```python
from build123d import *

# Parameters (mm, degrees)
F0_R     = 20.05
F1_DEPTH = 3.1
F2_R     = 10.05
F3_DEPTH = 2
F4_R     = 0.5
F5_R     = 2.5
F6_DEPTH = 3.1010001
F7_W     = 1
F7_H     = 5
F8_DEPTH = 3.1010001


with BuildPart() as f1:
    # F0 (on Top) → F1 (new body)
    with BuildSketch(Plane.XY):
        Circle(F0_R)
    extrude(amount=F1_DEPTH)

    # F2 (on face) → F3 (cut)
    with BuildSketch(Plane.XY.offset(3.1)):
        with Locations((5, 0)):
            Circle(F2_R)
    extrude(amount=-F3_DEPTH, mode=Mode.SUBTRACT)

    # F4
    f4_edges = [f1.edges().sort_by_distance(p)[0] for p in [
        (-20.05, 0, 3.1),
        (-5.05, 0, 3.1),
        (-20.05, 0, 0),
    ]]
    fillet(f4_edges, radius=F4_R)

    # F5 (on face) → F6 (cut, through all)
    with BuildSketch(Plane(origin=(0, 0, 0), x_dir=(1, 0, 0), z_dir=(0, 0, -1))):
        Circle(F5_R)
    extrude(amount=-F6_DEPTH, mode=Mode.SUBTRACT)

    # F7 (on face) → F8 (cut, through all)
    with BuildSketch(Plane.XY.offset(3.1)):
        with Locations((0, 18.05)):
            Rectangle(F7_W, F7_H)
        with Locations((0, -18.05)):
            Rectangle(F7_W, F7_H)
    extrude(amount=-F8_DEPTH, mode=Mode.SUBTRACT)


solid = f1.part
```
CAD build for the part. Positions are in the model's coordinates, mm. A direction names the side the tool comes from. Round coordinates to 2 decimals unless told otherwise and drop trailing zeros. Order: outer loops, then holes, each group sorted by start corner. A loop starts at its lowest first (then second) coordinate and runs counter-clockwise, first axis right, second up.
Q1. Drop flat-ended pins along their axis: pin 1 (0.9 mm diameter, centred on y = -18, z = 2.5, fed in from -X); pin 2 (0.9 mm diameter, centred on y = 19, z = 1.5, fed in from +X); pin 3 (1 mm diameter, centred on x = 11, z = 0.5, fed in from -Y). Give the stop position or say it passes through.
Q2. Wall check: L1, parallel to X at y = 0, z = 0.8; L2, parallel to Y at x = 0, z = 0.3; L3, parallel to Y at x = 8, z = 1.2. Give the ranges that are in metal, low to high.
Q3. Slice it at A-A (y = 0). Write the cut outline in (x, z), and give its area (3 significant figures).
Q4. Two-plate mould, pull along X, no slides. Class faces 5 (the flat face through (0, 15.55, 2)), 6 (the cylindrical face through (-20.045, 0.434, 1.535)), 7 (the cylindrical face through (20.045, -0.434, 1.535)): pulls with the +X half, pulls with the -X half, needs draft (parallel to the pull), parting line crosses it, or undercut.
Q5. Which spindle directions (+Z, -Z, +X, -X, +Y, -Y) get a long thin tool onto all of the face, cutting with end or side? Do faces 1 (the flat face through (-0.5, 18, 2)), 2 (the flat face through (4, 0, 0)), 3 (the flat face through (5, 0, 1.1)), 4 (the flat face through (0.5, -18, 2)). Say none if no direction does.
Results below:
1. pin 1: stops at x = -9.7
1. pin 2: stops at x = 7.61
1. pin 3: stops at y = -17.08
2. L1: x = -20.05 to -2.5, 2.5 to 20.05
2. L2: y = -15.55 to -2.5, 2.5 to 15.55
2. L3: y = -18.38 to -9.59, 9.59 to 18.38
3. outline: (-20.05, 0.5) arc R0.5 ccw to (-19.55, 0) - (-2.5, 0) - (-2.5, 1.1) - (-5.05, 1.1) - (-5.05, 2.6) arc R0.5 ccw to (-5.55, 3.1) - (-19.55, 3.1) arc R0.5 ccw to (-20.05, 2.6) - close; (2.5, 0) - (19.55, 0) arc R0.5 ccw to (20.05, 0.5) - (20.05, 2.6) arc R0.5 ccw to (19.55, 3.1) - (15.55, 3.1) arc R0.5 ccw to (15.05, 2.6) - (15.05, 1.1) - (2.5, 1.1) - close
3. area: 78.3 mm2
4. face 5: undercut
4. face 6: pulls with the -X half
4. face 7: pulls with the +X half
5. face 1: +Z, -Z, +Y
5. face 2: -Z, +X, -X, +Y, -Y
5. face 3: +Z
5. face 4: +Z, -Z, -Y
